Can you work these out from the model? Positions are in its coordinate system, mm. Face numbers are marked on the shaded views. A direction names the side the tool comes from. Coordinates: 2 decimals unless noted, no trailing zeros. Loops run counter-clockwise (first coordinate to the right, second up) from the corner with the lowest first, then second, coordinate; pieces in that order, holes last. Notation, with made-up numbers: (55, 77) -> (85, 77) arc R8 cw to (85, 88) -> close; hole circle Ø8 at (-23, 56.5). An arc over 180 degrees is marked (long way). Put each result on its own line as item: value. Start each with the question number.
Item 1: If we section it at B-B on x = -66: Please give me the cut outline in (y, z), plus the area to 3 significant figures.
Item 2: If we section it at A-A on z = -2.75: Please give me the cut outline in (x, y).
Item 3: Please list where these lines run through material, in increasing order: L1, parallel to X at y = 33, z = -6.25; L2, parallel to Y at x = -26, z = 11; L3, parallel to X at y = 8, z = 13. Write a range as from..to.
Item 4: If we section it at C-C on x = -10: Please give me the cut outline in (y, z), plus the area to 3 significant figures.
Item 5: We'd pull the mould along Y, two halves only. Please class the marked faces 4, 5 and 6: pulls with the +Y half, pulls with the -Y half, needs draft (parallel to the pull), parting line crosses it, or undercut.
Item 6: For the marked faces 1, 2 and 3, which set-ups out of +Z, -Z, +X, -X, +Y, -Y let a thin tool reach every point of the face, with its end or its side?
Item 7: If we section it at D-D on x = -42: Please give me the cut outline in (y, z).
Item 8: Will these pins go through, and if not, where does the flat tip stop? P1, Ø8, axis at x = -36, y = 4, coming from the -Z side; P2, Ø4.5, axis at x = -64, z = 1, coming from the -Y side; P3, Ø0.8, axis at x = -65.5, y = -1.5, coming from the -Z side.
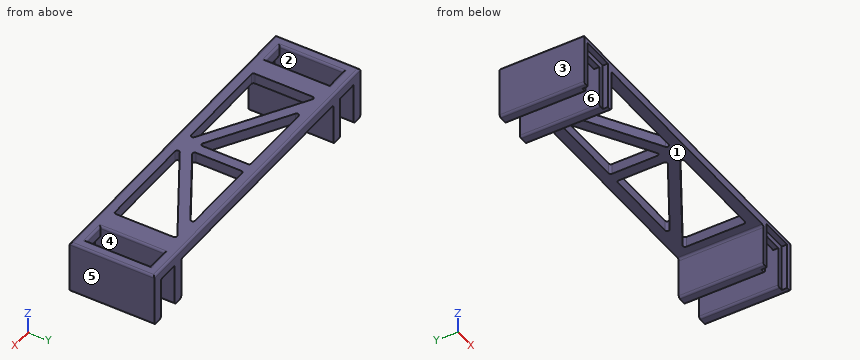
```python
from build123d import *

# Parameters (mm, degrees)
BOSS_EXTRUDE2_DEPTH     = 37.5
BOSS_EXTRUDE3_DEPTH     = 2.5
CUT_EXTRUDE1_DEPTH      = 89.519898893
CUT_EXTRUDE1_DEPTH_BACK = 89.519898893
SKETCH8_W               = 10.3
SKETCH8_H               = 30
CUT_EXTRUDE3_DEPTH      = 89.519898893
FILLET1_R               = 1


with BuildPart() as part:
    # Sketch2 → Boss-Extrude2 (new body)
    with BuildSketch(Plane(origin=(0, 0, 0), x_dir=(1, 0, 0), z_dir=(0, 1, 0))):
        Polygon((77.65, -15), (77.65, 10), (72.65, 10), (72.65, -10), (62.35, -10), (62.35, 10), (57.35, 10), (57.35, -10), (-57.35, -10), (-57.35, 10), (-62.35, 10), (-62.35, -10), (-72.65, -10), (-72.65, 10), (-77.65, 10), (-77.65, -15), align=None)
    extrude(amount=BOSS_EXTRUDE2_DEPTH)

    # Sketch3 → Boss-Extrude3 (add)
    with BuildSketch(Plane(origin=(0, 0, 0), x_dir=(1, 0, 0), z_dir=(0, 1, 0))):
        Polygon((77.65, 10), (77.65, -15), (-77.65, -15), (-77.65, 10), (-75.15, 10), (-75.15, -12.5), (-59.85, -12.5), (-59.85, 10), (-57.35, 10), (-57.35, -10), (57.35, -10), (57.35, 10), (59.85, 10), (59.85, -12.5), (75.15, -12.5), (75.15, 10), align=None)
    extrude(amount=-BOSS_EXTRUDE3_DEPTH)

    # Sketch4 → Cut-Extrude1 (cut, two sides: drawn at the far end of the back side and taken through both)
    with BuildSketch(Plane(origin=(0, 0, 10), x_dir=(-1, 0, 0), z_dir=(0, 0, -1)).offset(-CUT_EXTRUDE1_DEPTH_BACK)):
        Polygon((52.35, 2.5), (52.35, 32.5), (2.5, 2.5), align=None)
        Polygon((-2.5, 2.5), (-52.35, 2.5), (-52.35, 32.5), align=None)
        Polygon((42.653175634, 32.5), (2.5, 8.335601424), (2.5, 32.5), align=None)
        Polygon((-2.5, 8.335601424), (-2.5, 32.5), (-42.653175634, 32.5), align=None)
    extrude(amount=CUT_EXTRUDE1_DEPTH + CUT_EXTRUDE1_DEPTH_BACK, mode=Mode.SUBTRACT)

    # Sketch8 → Cut-Extrude3 (cut, through all)
    with BuildSketch(Plane(origin=(0, 0, 10), x_dir=(-1, 0, 0), z_dir=(0, 0, -1))):
        with Locations((67.5, 17.5)):
            Rectangle(SKETCH8_W, SKETCH8_H)
        with Locations((-67.5, 17.5)):
            Rectangle(SKETCH8_W, SKETCH8_H)
    extrude(amount=-CUT_EXTRUDE3_DEPTH, mode=Mode.SUBTRACT)

    # Fillet1
    fillet1_edges = [part.edges().sort_by_distance(p)[0] for p in [
        (2.5, 8.335601424, 12.5),
        (42.653175634, 32.5, 12.5),
        (2.5, 32.5, 12.5),
        (-52.35, 2.5, 12.5),
        (-2.5, 2.5, 12.5),
        (-52.35, 32.5, 12.5),
        (-2.5, 32.5, 12.5),
        (-42.653175634, 32.5, 12.5),
        (-2.5, 8.335601424, 12.5),
        (52.35, 32.5, 12.5),
        (2.5, 2.5, 12.5),
        (52.35, 2.5, 12.5),
        (-72.65, 17.5, 15),
        (-67.5, 2.5, 15),
        (-62.35, 17.5, 15),
        (-67.5, 32.5, 15),
        (62.35, 17.5, 15),
        (67.5, 2.5, 15),
        (72.65, 17.5, 15),
        (67.5, 32.5, 15),
        (0, 37.5, 15),
        (-62.35, 18.75, -10),
        (-57.35, 17.5, -10),
        (-57.35, 17.5, 10),
        (57.35, 17.5, 10),
        (57.35, 17.5, -10),
        (62.35, 18.75, -10),
        (72.65, 18.75, -10),
        (77.65, 17.5, -10),
        (77.65, 17.5, 15),
        (-77.65, 17.5, 15),
        (-77.65, 17.5, -10),
        (-72.65, 18.75, -10),
        (0, -2.5, 15),
    ]]
    fillet(fillet1_edges, radius=FILLET1_R)


solid = part.part
```
Solutions:
1. outline: (-2.5, 12.5) -> (0, 12.5) -> (0, 10) -> (2.5, 10) -> (2.5, 14) arc R1 ccw to (1.5, 15) -> (-1.5, 15) arc R1 ccw to (-2.5, 14) -> close; (32.5, 10) -> (37.5, 10) -> (37.5, 14) arc R1 ccw to (36.5, 15) -> (33.5, 15) arc R1 ccw to (32.5, 14) -> close
1. area: 42.9 mm^2
2. outline: (-77.65, -2.5) -> (-75.15, -2.5) -> (-75.15, 0) -> (-72.65, 0) -> (-72.65, 37.5) -> (-77.65, 37.5) -> close; (-62.35, 0) -> (-59.85, 0) -> (-59.85, -2.5) -> (-57.35, -2.5) -> (-57.35, 37.5) -> (-62.35, 37.5) -> close; (57.35, -2.5) -> (59.85, -2.5) -> (59.85, 0) -> (62.35, 0) -> (62.35, 37.5) -> (57.35, 37.5) -> close; (72.65, 0) -> (75.15, 0) -> (75.15, -2.5) -> (77.65, -2.5) -> (77.65, 37.5) -> (72.65, 37.5) -> close
3. L1: -77.65..-72.65, -62.35..-57.35, 57.35..62.35, 72.65..77.65
3. L2: -2.5..2.5, 16.64..22.48, 32.5..37.5
3. L3: -77.65..-72.65, -62.35..-52.35, -11.64..11.64, 52.35..62.35, 72.65..77.65
4. outline: (-2.5, 10) -> (2.5, 10) -> (2.5, 15) -> (-1.5, 15) arc R1 ccw to (-2.5, 14) -> close; (7.01, 10) -> (12.85, 10) -> (12.85, 15) -> (7.01, 15) -> close; (32.5, 10) -> (37.5, 10) -> (37.5, 14) arc R1 ccw to (36.5, 15) -> (32.5, 15) -> close
4. area: 78.7 mm^2
5. face 4: undercut
5. face 5: needs draft
5. face 6: undercut
6. face 1: -Z, +Y, -Y
6. face 2: -Z
6. face 3: +Z, -Z, -X, +Y, -Y
7. outline: (-2.5, 10) -> (2.5, 10) -> (2.5, 15) -> (-1.5, 15) arc R1 ccw to (-2.5, 14) -> close; (26.27, 10) -> (37.5, 10) -> (37.5, 14) arc R1 ccw to (36.5, 15) -> (26.27, 15) -> close
8. P1: z = 10
8. P2: y = 0
8. P3: z = 12.5
